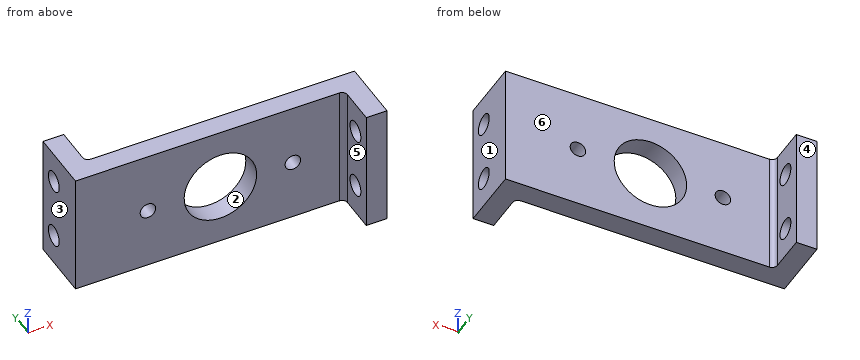
```python
from build123d import *

# Parameters (mm, degrees)
SKETCH1_W               = 177.8
SKETCH1_H               = 76.2
SKETCH1_R               = 22.225
SKETCH1_R_2             = 4.7625
BOSS_EXTRUDE1_DEPTH     = 12.7
SKETCH2_W               = 12.7
SKETCH2_H               = 76.2
BOSS_EXTRUDE2_DEPTH     = 25.4
SKETCH3_W               = 12.7
SKETCH3_H               = 76.2
BOSS_EXTRUDE3_DEPTH     = 25.4
CUT_EXTRUDE1_DEPTH      = 174.669888006
CUT_EXTRUDE1_DEPTH_BACK = 174.669888006
SKETCH4_R               = 6.35
FILLET1_R               = 3.175


with BuildPart() as part:
    # Sketch1 → Boss-Extrude1 (new body)
    with BuildSketch(Plane(origin=(0, 0, 0), x_dir=(1, 0, 0), z_dir=(0, 1, 0))):
        Rectangle(SKETCH1_W, SKETCH1_H)
        with Locations(Location((0, 0, 0), (0, 0, 270))):
            Circle(SKETCH1_R, mode=Mode.SUBTRACT)
        with Locations(Location((-44.45, 0, 0), (0, 0, 270))):
            Circle(SKETCH1_R_2, mode=Mode.SUBTRACT)
        with Locations(Location((44.45, 0, 0), (0, 0, 270))):
            Circle(SKETCH1_R_2, mode=Mode.SUBTRACT)
    extrude(amount=BOSS_EXTRUDE1_DEPTH)

    # Sketch2 → Boss-Extrude2 (add)
    with BuildSketch(Plane(origin=(0, 12.7, 0), x_dir=(1, 0, 0), z_dir=(0, 1, 0))):
        with Locations((-82.55, 0)):
            Rectangle(SKETCH2_W, SKETCH2_H)
    extrude(amount=BOSS_EXTRUDE2_DEPTH)

    # Sketch3 → Boss-Extrude3 (add)
    with BuildSketch(Plane.XZ):
        with Locations((82.55, 0)):
            Rectangle(SKETCH3_W, SKETCH3_H)
    extrude(amount=BOSS_EXTRUDE3_DEPTH)

    # Sketch4 → Cut-Extrude1 (cut, two sides: drawn at the far end of the back side and taken through both)
    with BuildSketch(Plane(origin=(-76.2, 0, 0), x_dir=(0, 0, -1), z_dir=(1, 0, 0)).offset(-CUT_EXTRUDE1_DEPTH_BACK)):
        with Locations((-19.05, 25.4)):
            Circle(SKETCH4_R)
        with Locations((19.05, 25.4)):
            Circle(SKETCH4_R)
        with Locations((-19.05, -12.7)):
            Circle(SKETCH4_R)
        with Locations((19.05, -12.7)):
            Circle(SKETCH4_R)
    extrude(amount=CUT_EXTRUDE1_DEPTH + CUT_EXTRUDE1_DEPTH_BACK, mode=Mode.SUBTRACT)

    # Fillet1
    fillet1_edges = [part.edges().sort_by_distance(p)[0] for p in [
        (-76.2, 12.7, 0),
        (76.2, 0, 0),
    ]]
    fillet(fillet1_edges, radius=FILLET1_R)


solid = part.part
```
Work out the finished part from the listing and answer in its coordinate system (mm). Face numbers are marked on the shaded views. A direction names the side the tool comes from. Give positions to 0.01 mm unless a question says otherwise; leave off trailing zeros. Order: outer loops, then holes, each group sorted by start corner. A loop starts at its lowest first (then second) coordinate and runs counter-clockwise, first axis right, second up.
1. Section A-A, the plane x = 44.45 is taken. Determine the outline of the cut face in (y, z).
Result sheet:
outline: (0, -38.1) - (12.7, -38.1) - (12.7, -4.76) - (0, -4.76) - close; (0, 4.76) - (12.7, 4.76) - (12.7, 38.1) - (0, 38.1) - close
2. Each of these flat-tipped pins is pushed along its axis until it touches: P1, Ø6.5, axis at y = 27.5, z = -10.5, coming from the +X side; P2, Ø11, axis at x = -44.45, z = 0, coming from the -Y side; P3, Ø6.5, axis at y = -10, z = -2, coming from the -X side. Where does it stop, or does it pass through?
Result sheet:
P1: stops at x = -76.2
P2: stops at y = 0
P3: stops at x = 76.2
3. Section C-C, the plane y = -12.7 is taken. Determine the outline of the cut face in (x, z), and give its area (3 significant figures).
Result sheet:
outline: (76.2, -38.1) - (88.9, -38.1) - (88.9, -25.4) - (76.2, -25.4) - close; (76.2, -12.7) - (88.9, -12.7) - (88.9, 12.7) - (76.2, 12.7) - close; (76.2, 25.4) - (88.9, 25.4) - (88.9, 38.1) - (76.2, 38.1) - close
area: 645 mm2
4. Section B-B, the plane z = -3 is taken. Determine the outline of the cut face in (x, y) (3 decimals).
Result sheet:
outline: (-88.9, 0) - (-48.149, 0) - (-48.149, 12.7) - (-73.025, 12.7) arc R3.175 cw to (-76.2, 15.875) - (-76.2, 38.1) - (-88.9, 38.1) - close; (-40.751, 0) - (-22.022, 0) - (-22.022, 12.7) - (-40.751, 12.7) - close; (22.022, 0) - (40.751, 0) - (40.751, 12.7) - (22.022, 12.7) - close; (48.149, 0) - (73.025, 0) arc R3.175 cw to (76.2, -3.175) - (76.2, -25.4) - (88.9, -25.4) - (88.9, 12.7) - (48.149, 12.7) - close
5. The mould has two halves that part along X. Classify the marked faces 1, 2 and 3: released by +X, released by -X, zero draft, split by the parting line, or undercut.
Result sheet:
face 1: released by +X
face 2: undercut
face 3: released by -X
6. For the marked faces 4, 5 and 6, determine the directions among +Z, -Z, +X, -X, +Y, -Y from which every point of the face is accessible in a straight line to the end or side of a thin tool.
Result sheet:
face 4: +Z, -Z, +X, -X, +Y
face 5: +Z, -Z, -X, -Y
face 6: +Z, -Z, +X, +Y
7. Straight lines are drawn through the part: L1, parallel to X at y = 7, z = 0 (1 decimal); L2, parallel to Y at x = -80.75, z = -19.05; L3, parallel to X at y = -6, z = 19. For each, find the intervals that lie inside material, in ascending order.
Result sheet:
L1: x = -88.9 to -49.2, -39.7 to -22.2, 22.2 to 39.7, 49.2 to 88.9
L2: y = 0 to 19.05, 31.75 to 38.1
L3: x = 76.2 to 88.9
8. Section D-D, the plane y = 9 is taken. Give the number of separate pieces and of enclosed holes in the cut face, and give its area (3 significant figures).
Result sheet:
separate pieces: 1
enclosed holes: 3
area: 11,900 mm2
